Here's the drawing with two shaded views (mm, measured from the low corner). I have some questions. A direction names the side the tool comes from. Coordinates: 2 decimals unless noted, no trailing zeros. Write each loop counter-clockwise with the first axis right and the second up, starting at its lowest first coordinate (ties: lowest second). Pieces come first, ordered by that corner, then holes.
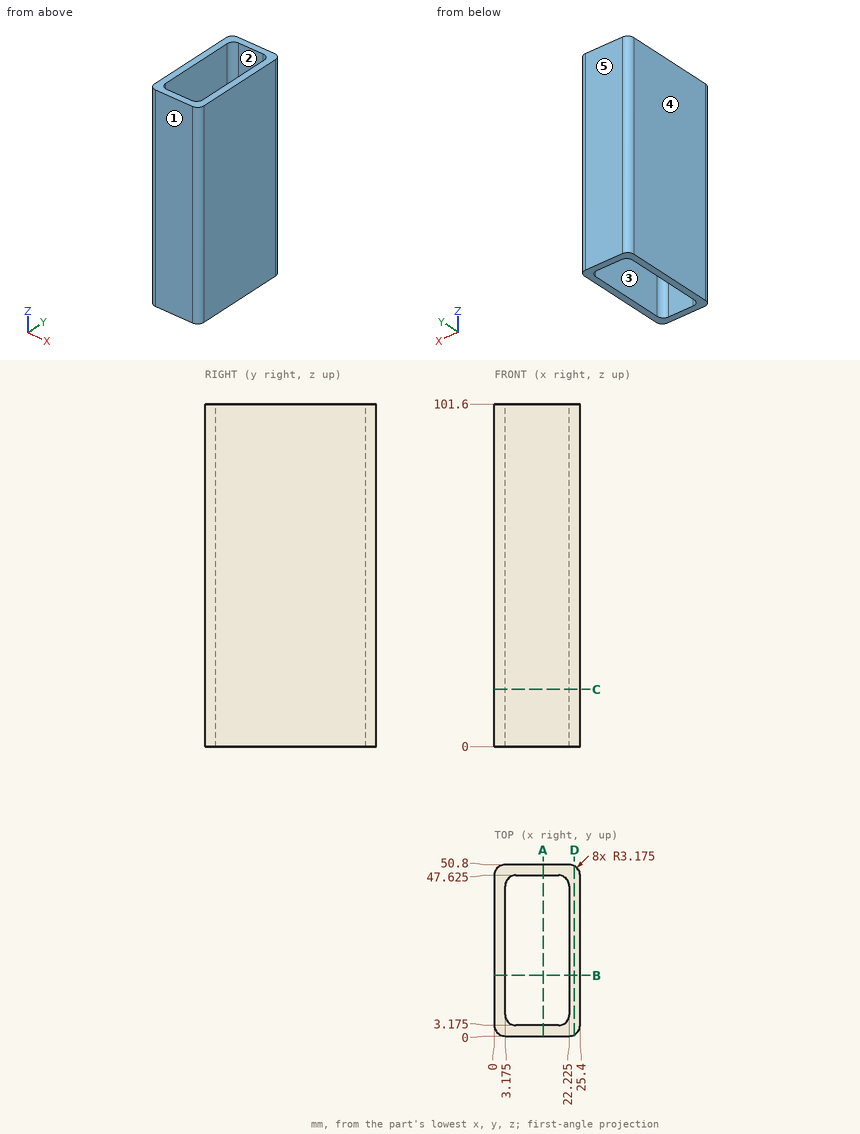
Item 1: I want a section at D-D, the plane x = 23.75. List the corners of the cut face in (y, z) for me.
Item 2: I want a section at C-C, the plane z = 17. List the corners of the cut face in (x, y) for me (3 decimals).
Item 3: If I drill on line 1 along X through (y, z) = (44, 20) (3 decimals); line 2 along Y through (x, z) = (16, 48) (3 decimals); line 3 along Y through (x, z) = (5, 11.5), over which ranges is the centre line in solid material (lowest first)?
Item 4: If we mould it in two halves opening along X, with no side actions, what happens to the marked faces 3, 4 and 5? For each: released by +X, released by -X, zero draft, split by the parting line, or undercut.
Item 5: I want a section at B-B, the plane y = 18. List the corners of the cut face in (x, z) for me (3 decimals).
Item 6: Which directions (+Z, -Z, +X, -X, +Y, -Y) give clear straight access to the entire face, cutting with the end or side of a thin tool? Please do the marked faces 1 and 2.
Item 7: I want a section at A-A, the plane x = 14.5. List the corners of the cut face in (y, z) for me (3 decimals).
Taken from the geometry:
1. outline: (0.39, 0) - (50.41, 0) - (50.41, 101.6) - (0.39, 101.6) - close
2. outline: (0, 3.175) arc R3.175 ccw to (3.175, 0) - (22.225, 0) arc R3.175 ccw to (25.4, 3.175) - (25.4, 47.625) arc R3.175 ccw to (22.225, 50.8) - (3.175, 50.8) arc R3.175 ccw to (0, 47.625) - close; hole (3.175, 6.35) arc R3.175 ccw to (6.35, 3.175) - (19.05, 3.175) arc R3.175 ccw to (22.225, 6.35) - (22.225, 44.45) arc R3.175 ccw to (19.05, 47.625) - (6.35, 47.625) arc R3.175 ccw to (3.175, 44.45) - close
3. line 1: x = 0 to 3.175, 22.225 to 25.4
3. line 2: y = 0 to 3.175, 47.625 to 50.8
3. line 3: y = 0 to 3.48, 47.32 to 50.8
4. face 3: undercut
4. face 4: released by -X
4. face 5: zero draft
5. outline: (0, 0) - (3.175, 0) - (3.175, 101.6) - (0, 101.6) - close; (22.225, 0) - (25.4, 0) - (25.4, 101.6) - (22.225, 101.6) - close
6. face 1: +Z, -Z, +X, -X, -Y
6. face 2: +Z, -Z
7. outline: (0, 0) - (3.175, 0) - (3.175, 101.6) - (0, 101.6) - close; (47.625, 0) - (50.8, 0) - (50.8, 101.6) - (47.625, 101.6) - close
